Could you check a few things on this model? Use its own coordinates, in mm. A direction names the side the tool comes from. Give positions to 0.01 mm unless a question says otherwise; leave off trailing zeros. Order: outer loops, then holes, each group sorted by start corner. A loop starts at its lowest first (then second) coordinate and runs counter-clockwise, first axis right, second up. Notation, with made-up numbers: M 23,-26 L 27,-26 A20 cw 27,6 Z; hole C -14.5,81 d8. An arc over 180 degrees is marked long. Use a Markdown table: item, result. Add a question column.
Item 1: Suppose I cut it at C-C on x = -2.5. Write out the boundary of the cut face in (y, z).
Item 2: Suppose I cut it at B-B on y = -11. Write out the boundary of the cut face in (x, z), plus the area to 3 significant figures.
Item 3: Suppose I cut it at A-A on z = 9. Write out the boundary of the cut face in (x, y).
Item 4: If I drill on L1, parallel to X at y = 17, z = 11.25; L2, parallel to Y at x = 10.5, z = 11; L3, parallel to Z at x = 1.5, y = -8, over which ranges is the centre line in solid material (lowest first)? Write a range as from..to.
Item 5: If we mould it in two halves opening along X, with no side actions, what happens to faces 4 (the face through (25.1, -29.6, 0.7)), 5 (the face through (-22.991, 28.574, 10.62)), 6 (the face through (-22.995, 0, 11))? For each: released by +X, released by -X, zero draft, split by the parting line, or undercut.
Item 6: I'm going to push flat-ended pins straight in: pin 1 Ø9 at (y, z) = (0.5, 9.5) entering from -X; pin 2 Ø6 at (x, z) = (17.5, 14.5) entering from -Y; pin 3 Ø8 at (x, z) = (1.5, 13) entering from +Y. Where does each tip first touch, or does it pass through?
Item 7: For faces 1 (the face through (22.952, 27.502, 10.62)), 2 (the face through (-23.069, -28.496, 10.62)), 3 (the face through (24.001, -28.574, 10.62)), which set-ups out of +Z, -Z, +X, -X, +Y, -Y let a thin tool reach every point of the face, with its end or its side?
from build123d import *

# Parameters (mm, degrees)
F1_DEPTH = 1.5
F2_DEPTH = 20


with BuildPart() as f1:
    # F0 (on Top) → F1 (new body)
    with BuildSketch(Plane.XY):
        with BuildLine():
            ThreePointArc((-19.49504, 31.5), (-24.091234, 29.596194), (-25.99504, 25))
            Line((-25.99504, 25), (-25.99504, -25))
            ThreePointArc((-25.99504, -25), (-24.091234, -29.596194), (-19.49504, -31.5))
            Line((-19.49504, -31.5), (20.50496, -31.5))
            ThreePointArc((20.50496, -31.5), (25.101155, -29.596194), (27.00496, -25))
            Line((27.00496, -25), (27.00496, 25))
            ThreePointArc((27.00496, 25), (25.101155, 29.596194), (20.50496, 31.5))
            Line((20.50496, 31.5), (-19.49504, 31.5))
        make_face()
        with BuildLine():
            Line((-19.49504, 30), (20.50496, 30))
            ThreePointArc((20.50496, 30), (24.040494, 28.535534), (25.50496, 25))
            Line((25.50496, 25), (25.50496, -25))
            ThreePointArc((25.50496, -25), (24.040494, -28.535534), (20.50496, -30))
            Line((20.50496, -30), (-19.49504, -30))
            ThreePointArc((-19.49504, -30), (-23.030573, -28.535534), (-24.49504, -25))
            Line((-24.49504, -25), (-24.49504, 25))
            ThreePointArc((-24.49504, 25), (-23.030573, 28.535534), (-19.49504, 30))
        make_face(mode=Mode.SUBTRACT)
        with BuildLine():
            ThreePointArc((25.50496, 25), (24.040494, 28.535534), (20.50496, 30))
            Line((20.50496, 30), (-19.49504, 30))
            ThreePointArc((-19.49504, 30), (-23.030573, 28.535534), (-24.49504, 25))
            Line((-24.49504, 25), (-24.49504, -25))
            ThreePointArc((-24.49504, -25), (-23.030573, -28.535534), (-19.49504, -30))
            Line((-19.49504, -30), (20.50496, -30))
            ThreePointArc((20.50496, -30), (24.040494, -28.535534), (25.50496, -25))
            Line((25.50496, -25), (25.50496, 25))
        make_face()
        with BuildLine():
            ThreePointArc((20.50496, 28.5), (22.979834, 27.474874), (24.00496, 25))
            Line((24.00496, 25), (24.00496, -25))
            ThreePointArc((24.00496, -25), (22.979834, -27.474874), (20.50496, -28.5))
            Line((20.50496, -28.5), (-19.49504, -28.5))
            ThreePointArc((-19.49504, -28.5), (-21.969913, -27.474874), (-22.99504, -25))
            Line((-22.99504, -25), (-22.99504, 25))
            ThreePointArc((-22.99504, 25), (-21.969913, 27.474874), (-19.49504, 28.5))
            Line((-19.49504, 28.5), (20.50496, 28.5))
        make_face(mode=Mode.SUBTRACT)
        with BuildLine():
            Line((24.00496, -25), (24.00496, 25))
            ThreePointArc((24.00496, 25), (22.979834, 27.474874), (20.50496, 28.5))
            Line((20.50496, 28.5), (-19.49504, 28.5))
            ThreePointArc((-19.49504, 28.5), (-21.969913, 27.474874), (-22.99504, 25))
            Line((-22.99504, 25), (-22.99504, -25))
            ThreePointArc((-22.99504, -25), (-21.969913, -27.474874), (-19.49504, -28.5))
            Line((-19.49504, -28.5), (20.50496, -28.5))
            ThreePointArc((20.50496, -28.5), (22.979834, -27.474874), (24.00496, -25))
        make_face()
    extrude(amount=F1_DEPTH)

    # F0 (on Top) → F2 (join)
    with BuildSketch(Plane.XY):
        with BuildLine():
            ThreePointArc((25.50496, 25), (24.040494, 28.535534), (20.50496, 30))
            Line((20.50496, 30), (-19.49504, 30))
            ThreePointArc((-19.49504, 30), (-23.030573, 28.535534), (-24.49504, 25))
            Line((-24.49504, 25), (-24.49504, -25))
            ThreePointArc((-24.49504, -25), (-23.030573, -28.535534), (-19.49504, -30))
            Line((-19.49504, -30), (20.50496, -30))
            ThreePointArc((20.50496, -30), (24.040494, -28.535534), (25.50496, -25))
            Line((25.50496, -25), (25.50496, 25))
        make_face()
        with BuildLine():
            ThreePointArc((20.50496, 28.5), (22.979834, 27.474874), (24.00496, 25))
            Line((24.00496, 25), (24.00496, -25))
            ThreePointArc((24.00496, -25), (22.979834, -27.474874), (20.50496, -28.5))
            Line((20.50496, -28.5), (-19.49504, -28.5))
            ThreePointArc((-19.49504, -28.5), (-21.969913, -27.474874), (-22.99504, -25))
            Line((-22.99504, -25), (-22.99504, 25))
            ThreePointArc((-22.99504, 25), (-21.969913, 27.474874), (-19.49504, 28.5))
            Line((-19.49504, 28.5), (20.50496, 28.5))
        make_face(mode=Mode.SUBTRACT)
    extrude(amount=F2_DEPTH)


solid = f1.part
Findings below:
| question | item | result |
|---|---|---|
| 1 | outline | M -31.5,0 L 31.5,0 L 31.5,1.5 L 30,1.5 L 30,20 L 28.5,20 L 28.5,1.5 L -28.5,1.5 L -28.5,20 L -30,20 L -30,1.5 L -31.5,1.5 Z |
| 2 | outline | M -26,0 L 27,0 L 27,1.5 L 25.5,1.5 L 25.5,20 L 24,20 L 24,1.5 L -23,1.5 L -23,20 L -24.5,20 L -24.5,1.5 L -26,1.5 Z |
| 2 | area | 135 mm^2 |
| 3 | outline | M -24.5,-25 A5 ccw -19.5,-30 L 20.5,-30 A5 ccw 25.5,-25 L 25.5,25 A5 ccw 20.5,30 L -19.5,30 A5 ccw -24.5,25 Z; hole M -23,-25 A3.5 ccw -19.5,-28.5 L 20.5,-28.5 A3.5 ccw 24,-25 L 24,25 A3.5 ccw 20.5,28.5 L -19.5,28.5 A3.5 ccw -23,25 Z |
| 4 | L1 | x = -24.5..-23, 24..25.5 |
| 4 | L2 | y = -30..-28.5, 28.5..30 |
| 4 | L3 | z = 0..1.5 |
| 5 | face 4 | released by +X |
| 5 | face 5 | released by -X |
| 5 | face 6 | undercut |
| 6 | pin 1 | stops at x = -24.5 |
| 6 | pin 2 | stops at y = -30 |
| 6 | pin 3 | stops at y = 30 |
| 7 | face 1 | +Z |
| 7 | face 2 | +Z, -X, -Y |
| 7 | face 3 | +Z, +X, -Y |
